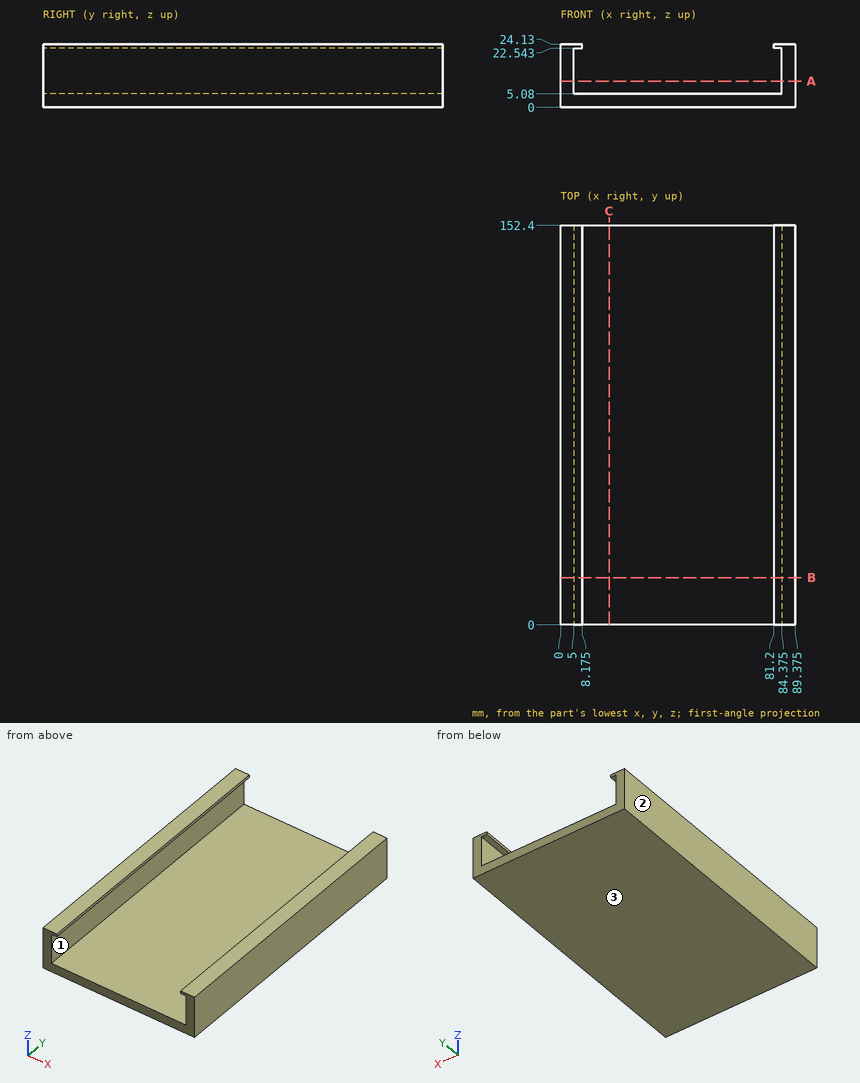
Input: dimensioned drawing with shaded views. Units: mm. Origin: part minimum x, y, z. Give positions to 0.01 mm unless a question says otherwise; leave off trailing zeros. Loops run counter-clockwise (first coordinate to the right, second up) from the corner with the lowest first, then second, coordinate; pieces in that order, holes last. Notation, with made-up numbers: (43, -2.5) -> (67, -2.5) arc R23 ccw to (67, 6.5) -> close; hole circle Ø5 at (-9, 67.25). An arc over 180 degrees is marked (long way). Return JSON: item names as keys, results as strings.
Item 1: Section B-B, the plane y = 18. Output: boundary loops of the cut face in (x, z) (1 decimal).
Filled in:
{"outline": "(0, 0) -> (89.4, 0) -> (89.4, 24.1) -> (81.2, 24.1) -> (81.2, 22.5) -> (84.4, 22.5) -> (84.4, 5.1) -> (5, 5.1) -> (5, 22.5) -> (8.2, 22.5) -> (8.2, 24.1) -> (0, 24.1) -> close"}
Item 2: Section A-A, the plane z = 10. Output: boundary loops of the cut face in (x, y) (1 decimal).
Filled in:
{"outline": "(0, 0) -> (5, 0) -> (5, 152.4) -> (0, 152.4) -> close; (84.4, 0) -> (89.4, 0) -> (89.4, 152.4) -> (84.4, 152.4) -> close"}
Item 3: Pin query (flat end, axial travel): P1, Ø4, axis at x = 15.5, y = 88.5, coming from the +Z side. Return the tip coordinate at first contact, or that it passes through.
Filled in:
{"P1": "z = 5.08"}
Item 4: Line query: line 1 (X direction, y = 100, z = 6.5) (1 decimal); line 2 (Z direction, x = 7.5, y = 75); line 3 (Z direction, x = 12, y = 50). Output: solid intervals per line, ascending.
Filled in:
{"line 1": "0 to 5, 84.4 to 89.4", "line 2": "0 to 5.08, 22.54 to 24.13", "line 3": "0 to 5.08"}
Item 5: Section C-C, the plane x = 18.5. Output: boundary loops of the cut face in (y, z).
Filled in:
{"outline": "(0, 0) -> (152.4, 0) -> (152.4, 5.08) -> (0, 5.08) -> close"}
Item 6: Mould query, pull axis X, two halves, no side actions, for the marked faces 1, 2 and 3. Classes: released by +X, released by -X, zero draft, split by the parting line, or undercut.
Filled in:
{"face 1": "undercut", "face 2": "released by -X", "face 3": "zero draft"}
